```python
from build123d import *

# Parameters (mm, degrees)
SKETCH_1_W                = 60
SKETCH_1_H                = 50
EXTRUDE_1_DEPTH           = 10
HOLE_WIZARD_2_D           = 8
HOLE_WIZARD_2_CSINK_D     = 8.2
HOLE_WIZARD_2_CSINK_ANGLE = 45
HOLE_WIZARD_3_D           = 5.2
SKETCH_8_W                = 80
SKETCH_8_H                = 60
EXTRUDE_2_DEPTH           = 10
SKETCH_11_W               = 20
SKETCH_11_H               = 7.6
CUT_EXTRUDE_1_DEPTH       = 21
SKETCH_12_W               = 20
SKETCH_12_H               = 5
EXTRUDE_4_DEPTH           = 30
HOLE_WIZARD_4_D           = 3.3
EXTRUDE_START             = -60
EXTRUDE_5_DEPTH           = 60
HOLE_WIZARD_5_D           = 8
HOLE_WIZARD_5_CSINK_D     = 8.5
HOLE_WIZARD_5_CSINK_ANGLE = 45
HOLE_WIZARD_6_D           = 8
HOLE_WIZARD_6_CSINK_D     = 8.2
HOLE_WIZARD_6_CSINK_ANGLE = 45
SKETCH_22_R               = 4.6
SKETCH_22_R_2             = 4.1
EXTRUDE_7_DEPTH           = 9.2


with BuildPart() as part:
    # 草图1 → 凸台-拉伸1 (new body)
    with BuildSketch(Plane.XY):
        Rectangle(SKETCH_1_W, SKETCH_1_H)
    extrude(amount=EXTRUDE_1_DEPTH)

    # 孔2 (through all)
    with Locations(Plane.XY.offset(10)):
        with Locations((20, 0), (-20, 0)):
            CounterSinkHole(HOLE_WIZARD_2_D / 2, HOLE_WIZARD_2_CSINK_D / 2, counter_sink_angle=HOLE_WIZARD_2_CSINK_ANGLE)

    # 孔3 (through all)
    with Locations(Plane(origin=(0, 0, 0), x_dir=(-1, 0, 0), z_dir=(0, 0, -1))):
        with Locations((0, 18), (0, -18)):
            Hole(HOLE_WIZARD_3_D / 2)

    # 草图8 → 凸台-拉伸2 (add)
    with BuildSketch(Plane.XZ.offset(25)):
        with Locations((10, 5)):
            Rectangle(SKETCH_8_W, SKETCH_8_H)
    extrude(amount=EXTRUDE_2_DEPTH)

    # 草图11 → 切除-拉伸1 (cut, symmetric)
    with BuildSketch(Plane.XY.offset(5)):
        with Locations((40, -31.2)):
            Rectangle(SKETCH_11_W, SKETCH_11_H)
    extrude(amount=CUT_EXTRUDE_1_DEPTH, both=True, mode=Mode.SUBTRACT)

    # 草图12 → 凸台-拉伸4 (add, symmetric)
    with BuildSketch(Plane.XY.offset(5)):
        with Locations((40, -22.5)):
            Rectangle(SKETCH_12_W, SKETCH_12_H)
    extrude(amount=EXTRUDE_4_DEPTH, both=True)

    # 孔4 (through all)
    with Locations(Plane(origin=(0, -20, 0), x_dir=(1, 0, 0), z_dir=(0, 1, 0))):
        with Locations((40, -15), (40, 5)):
            Hole(HOLE_WIZARD_4_D / 2)

    # 草图15 → 凸台-拉伸5 (add)
    with BuildSketch(Plane.XY.offset(35).offset(EXTRUDE_START)):
        Polygon((30, -20), (22.5, -25), (30, -25), align=None)
    extrude(amount=EXTRUDE_5_DEPTH)

    # 孔5 (through all)
    with Locations(Plane(origin=(0, 0, 0), x_dir=(-1, 0, 0), z_dir=(0, 0, -1))):
        with Locations((0, 0)):
            CounterSinkHole(HOLE_WIZARD_5_D / 2, HOLE_WIZARD_5_CSINK_D / 2, counter_sink_angle=HOLE_WIZARD_5_CSINK_ANGLE)

    # 孔6 (through all)
    with Locations(Plane(origin=(0, 0, 0), x_dir=(-1, 0, 0), z_dir=(0, 0, -1))):
        with Locations((-20, 0), (20, 0)):
            CounterSinkHole(HOLE_WIZARD_6_D / 2, HOLE_WIZARD_6_CSINK_D / 2, counter_sink_angle=HOLE_WIZARD_6_CSINK_ANGLE)

    # 草图22 → 凸台-拉伸7 (add)
    # profile 1 of 2: a face of its own
    with BuildSketch(Plane(origin=(0, 0, 0), x_dir=(-1, 0, 0), z_dir=(0, 0, -1))):
        with Locations((-20, 0)):
            Circle(SKETCH_22_R)
        with Locations((-20, 0)):
            Circle(SKETCH_22_R_2, mode=Mode.SUBTRACT)
    # profile 2 of 2: a face of its own
    with BuildSketch(Plane(origin=(0, 0, 0), x_dir=(-1, 0, 0), z_dir=(0, 0, -1))):
        with Locations((20, 0)):
            Circle(SKETCH_22_R)
        with Locations((20, 0)):
            Circle(SKETCH_22_R_2, mode=Mode.SUBTRACT)
    extrude(amount=EXTRUDE_7_DEPTH)


solid = part.part
```
The model under review builds one solid part; all positions refer to its coordinate system, in mm. A direction names the side the tool comes from. Round coordinates to 2 decimals unless told otherwise and drop trailing zeros. Loops run counter-clockwise (first coordinate to the right, second up) from the corner with the lowest first, then second, coordinate; pieces in that order, holes last.
1) Clearance check with flat-ended pins moving along their axes: P1, Ø12.5, axis at x = 8, z = -12, coming from the +Y side; P2, Ø10, axis at x = -2.5, y = -14, coming from the -Z side; P3, Ø4, axis at y = -30, z = -4.5, coming from the +X side; P4, Ø6.5, axis at x = 0, y = 0, coming from the -Z side. State where each tip first meets the part, or that it passes through.
Values follow:
P1: stops at y = -25
P2: stops at z = 0
P3: stops at x = 30
P4: passes through
2) Tool access review of faces 1 (the face through (1, -35, 5)), 2 (the face through (40, -31, 26)), 3 (the face through (-15.904, 0.18, -4.536)): name each direction out of +Z, -Z, +X, -X, +Y, -Y from which nothing blocks a thin tool from reaching the whole face with its end or side.
Values follow:
face 1: +Z, -Z, +X, -X, -Y
face 2: +X, -Y
face 3: -Z
3) Consider section A-A on z = 15. State the section outline as (x, y) points.
Values follow:
outline: (-30, -35) - (30, -35) - (30, -27.4) - (38.35, -27.4) - (38.35, -20) - (30, -20) - (22.5, -25) - (-30, -25) - close; (41.65, -27.4) - (50, -27.4) - (50, -20) - (41.65, -20) - close
4) Consider section B-B on y = 18. State the section outline as (x, z) points, then the cut area to 3 significant figures.
Values follow:
outline: (-30, 0) - (-2.6, 0) - (-2.6, 10) - (-30, 10) - close; (2.6, 0) - (30, 0) - (30, 10) - (2.6, 10) - close
area: 548 mm2
5) Consider section C-C on z = -5. State the section outline as (x, y) points.
Values follow:
outline: (-30, -35) - (30, -35) - (30, -27.4) - (38.35, -27.4) - (38.35, -20) - (30, -20) - (22.5, -25) - (-30, -25) - close; circle Ø9.2 at (-20, 0); circle Ø9.2 at (20, 0); (41.65, -27.4) - (50, -27.4) - (50, -20) - (41.65, -20) - close; hole circle Ø8.2 at (-20, 0); hole circle Ø8.2 at (20, 0)
6) Consider section D-D on x = 0. State the section outline as (y, z) points.
Values follow:
outline: (-35, -25) - (-25, -25) - (-25, 0) - (-20.6, 0) - (-20.6, 10) - (-25, 10) - (-25, 35) - (-35, 35) - close; (-15.4, 0) - (-4.25, 0) - (-4, 0.6) - (-4, 10) - (-15.4, 10) - close; (4, 0.6) - (4.25, 0) - (15.4, 0) - (15.4, 10) - (4, 10) - close; (20.6, 0) - (25, 0) - (25, 10) - (20.6, 10) - close
7) The part is to be moulded in two halves that separate along X. For faces 4 (the face through (0, 25, 5)), 5 (the face through (-0.338, 20.578, 5.07)), 6 (the face through (30, 2, 5)), say which applies: pulls with the +X half, pulls with the -X half, needs draft (parallel to the pull), parting line crosses it, or undercut.
Values follow:
face 4: needs draft
face 5: undercut
face 6: pulls with the +X half
8) Wall thickness on line 1 along Y through (x, z) = (0, 2.5); line 2 along X through (y, z) = (0, 7); line 3 along Z through (x, y) = (40, -24): over which ranges is each line inside the solid? List them lowest first.
Values follow:
line 1: y = -35 to -20.6, -15.4 to -4, 4 to 15.4, 20.6 to 25
line 2: x = -30 to -24, -16 to -4, 4 to 16, 24 to 30
line 3: z = -25 to -6.65, -3.35 to 13.35, 16.65 to 35
